```python
from build123d import *

# Parameters (mm, degrees)
F0_W     = 300
F0_H     = 10
F1_DEPTH = 200
F2_W     = 300
F2_H     = 5
F3_DEPTH = 90
F4_W     = 3
F4_H     = 75.580552
F5_DEPTH = 85
F6_R     = 3.189663
F7_DEPTH = 77


with BuildPart() as f1:
    # F0 (on Top) → F1 (new body)
    with BuildSketch(Plane.XY):
        with Locations((0, 15.697824)):
            Rectangle(F0_W, F0_H)
    extrude(amount=F1_DEPTH)

    # F2 (on face) → F3 (join)
    with BuildSketch(Plane.XZ.offset(-10.697824)):
        with Locations((0, 78.080552)):
            Rectangle(F2_W, F2_H)
    extrude(amount=F3_DEPTH)

    # F4 (on face) → F5 (join)
    with BuildSketch(Plane.XZ.offset(-10.697824)):
        with Locations((-148.5, 37.790276)):
            Rectangle(F4_W, F4_H)
    extrude(amount=F5_DEPTH)

    # F6 (on face) → F7 (join)
    with BuildSketch(Plane(origin=(0, 0, 75.580552), x_dir=(1, 0, 0), z_dir=(0, 0, -1))):
        with Locations((0, 72.494209)):
            Circle(F6_R)
    extrude(amount=F7_DEPTH)


solid = f1.part
```
Design review of the part built by this model. Coordinates are the model's own, in mm. A direction names the side the tool comes from. Give positions to 0.01 mm unless a question says otherwise; leave off trailing zeros. Loops run counter-clockwise (first coordinate to the right, second up) from the corner with the lowest first, then second, coordinate; pieces in that order, holes last. Notation, with made-up numbers: M 37.25,84.25 L 64.25,84.25 A15 ccw 64.25,92.25 Z; hole C 65,48 d4. An arc over 180 degrees is marked long. Return JSON: item names as keys, results as strings. Group by question number.
Item 1: We need section D-D (z = 175.5). Give the boundary of the cut face in (x, y).
Item 2: We need section B-B (z = 44.5). Give the boundary of the cut face in (x, y).
Item 3: We need section A-A (x = 25.5). Give the boundary of the cut face in (y, z), and give its area (3 significant figures).
Item 4: Insertion check: pin 1 Ø1 at (x, y) = (-4.5, -22) entering from -Z; pin 2 Ø5 at (x, y) = (-16.5, -8) entering from +Z; pin 3 Ø2 at (y, z) = (-40.5, 43) entering from +X. Each pin has a flat end and moves straight along its axis. Give the tip position at first contact, or say it passes through.
Item 5: Mouldability with a two-part tool opening along X and no side actions: class faces 3 (the flat face through (-2, 20.698, 99)), 4 (the flat face through (-150, -29, 54)), 5 (the cylindrical face through (-0.415, -75.657, 37.62)), 6 (the flat face through (150, 11, 92)) as released by +X, released by -X, zero draft, split by the parting line, or undercut.
Item 6: For probe 1 along Z at (x, y) = (-22.5, -68.5); probe 2 along X at (y, z) = (-23, 67); probe 3 along Y at (x, z) = (-106, 168), list the stretches that pass through material, from the lowest coordinate up.
Item 7: Tool access review of faces 1 (the flat face through (-2, -34, 80.581)), 2 (the flat face through (0, -73, -1.419)): name each direction out of +Z, -Z, +X, -X, +Y, -Y from which nothing blocks a thin tool from reaching the whole face with its end or side.
Item 8: We need section C-C (y = -50.5). Give the boundary of the cut face in (x, z).
Output:
{
 "1": {"outline": "M -150,10.7 L 150,10.7 L 150,20.7 L -150,20.7 Z"},
 "2": {"outline": "M -150,-74.3 L -147,-74.3 L -147,10.7 L 150,10.7 L 150,20.7 L -150,20.7 Z; C 0,-72.49 d6.38"},
 "3": {"outline": "M -79.3,75.58 L 10.7,75.58 L 10.7,0 L 20.7,0 L 20.7,200 L 10.7,200 L 10.7,80.58 L -79.3,80.58 Z", "area": "2,450 mm^2"},
 "4": {"pin 1": "stops at z = 75.58", "pin 2": "stops at z = 80.58", "pin 3": "stops at x = -147"},
 "5": {"face 3": "zero draft", "face 4": "released by -X", "face 5": "undercut", "face 6": "released by +X"},
 "6": {"probe 1": "z = 75.58 to 80.58", "probe 2": "x = -150 to -147", "probe 3": "y = 10.7 to 20.7"},
 "7": {"face 1": "+Z, +X, -X, -Y", "face 2": "-Z, +X, -X, +Y, -Y"},
 "8": {"outline": "M -150,0 L -147,0 L -147,75.58 L 150,75.58 L 150,80.58 L -150,80.58 Z"}
}
